The figure shows three views and two pictorial views of one solid part (mm, origin at its lowest corner). Answer the questions. A direction names the side the tool comes from. Round coordinates to 2 decimals unless told otherwise and drop trailing zeros. Order: outer loops, then holes, each group sorted by start corner. A loop starts at its lowest first (then second) coordinate and runs counter-clockwise, first axis right, second up. Notation, with made-up numbers: (1, 74.5) -> (30, 74.5) arc R17 ccw to (30, 96.5) -> close; hole circle Ø6 at (86.25, -21.75). An arc over 180 degrees is marked (long way). Return JSON: item names as keys, results as strings. Group by question number.
(1) Consider line 1 (Y direction, x = 1.7, z = 3.15); line 2 (X direction, y = 5.5, z = 2.1); line 3 (Z direction, x = 4.1, y = 3.75). Determine where each line is inside the solid, lowest interval first. Write a range as [from, to].
(2) Determine the mould class of the marked faces 1, 2 and 3 for opening direction Z: +Z half, -Z half, draft (parallel to the pull), parting line (faces both ways), or undercut.
(3) The part is cut by section D-D (y = 2). Determine the outline of the cut face in (x, z) (1 decimal).
(4) Which of the six approach directions +Z, -Z, +X, -X, +Y, -Y give full straight-line access (tool end or side, diameter ignored) to the marked faces 4, 5 and 6?
(5) The part is cut by section A-A (y = 5.75). Determine the outline of the cut face in (x, z) (1 decimal).
(6) Each of these flat-tipped pins is pushed along its axis until it touches: pin 1 (0.6 mm diameter, centred on y = 6, z = 1, fed in from +X); pin 2 (2 mm diameter, centred on x = 3, z = 2.5, fed in from +Y); pin 3 (1.4 mm diameter, centred on x = 1, y = 6, fed in from +Z); pin 4 (1.4 mm diameter, centred on y = 5.5, z = 4.5, fed in from +X) (1 decimal). Where does it stop, or does it pass through?
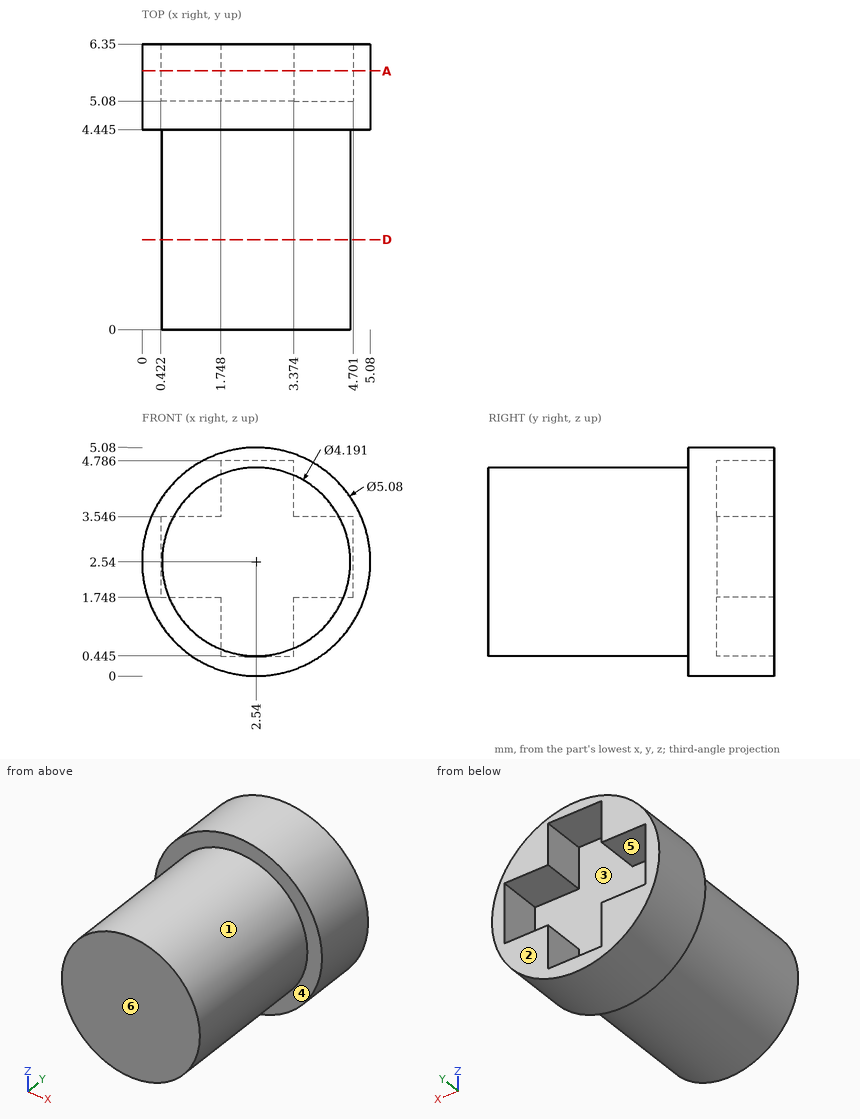
Answer below:
{
 "1": {"line 1": "y = [0, 5.08]", "line 2": "x = [0.04, 0.42], [4.7, 5.04]", "line 3": "z = [1.14, 3.94]"},
 "2": {"face 1": "parting line", "face 2": "draft", "face 3": "undercut"},
 "3": {"outline": "circle Ø4.2 at (2.5, 2.5)"},
 "4": {"face 4": "-Y", "face 5": "+Y", "face 6": "+Z, -Z, +X, -X, -Y"},
 "5": {"outline": "circle Ø5.1 at (2.5, 2.5); hole (0.4, 1.7) -> (1.7, 1.7) -> (1.7, 0.4) -> (3.4, 0.4) -> (3.4, 1.7) -> (4.7, 1.7) -> (4.7, 3.5) -> (3.4, 3.5) -> (3.4, 4.8) -> (1.7, 4.8) -> (1.7, 3.5) -> (0.4, 3.5) -> close"},
 "6": {"pin 1": "stops at x = 4.76", "pin 2": "stops at y = 6.35", "pin 3": "stops at z = 4.94", "pin 4": "stops at x = 4.7"}
}
